Autodesk Inventor part; units mm, degrees
ref_plane "YZ Plane" through (0, 0, 0) normal (1, 0, 0) x (0, 1, 0)
ref_plane "XZ Plane" through (0, 0, 0) normal (0, 1, 0) x (-1, 0, 0)
ref_plane "XY Plane" through (0, 0, 0) normal (0, 0, 1) x (1, 0, 0)
sketch "Sketch1" plane through (0, 0, 0) normal (0, 0, 1) x (1, 0, 0)
  circle A0 centre (0, 0) radius 235
  circle A1 centre (0, 0) radius 275
  circle A2 centre (0, 0) radius 255 construction
  line L0 (0, 275) -> (0, 235) construction
  point P0 (0, 255)
  dimension "d9" = 510
  dimension "d10" = 40
extrude "Plate1" add sketch "Sketch1" along normal blind 3
sketch "Sketch2" plane through (0, 0, 3) normal (0, 0, 1) x (1, 0, 0)
  circle A0 centre (0, 0) radius 235 construction
  circle A1 centre (0, 0) radius 275 construction
  line L0 (0, 275) -> (0, 235) construction
  circle A2 centre (0, 255) radius 9
  dimension "d3" = 18
extrude "Extrusion1" cut sketch "Sketch2" against normal through all
pattern_circular "Circular Pattern1" count 16 over 360 about axis through (0, 0, 0) along (0, 0, 1) of "Extrusion1"
equation "\"d9\" = Шпил_пласт_диам_центров"
equation "\"d10\" = Шпил_пласт_ширина"
equation "\"d2\" = Thickness"
equation "\"BendRadius\" = Thickness"
equation "\"BendReliefWidth\" = Thickness"
equation "\"BendReliefDepth\" = 0.5 * Thickness"
equation "\"CornerReliefSize\" = 4 * Thickness"
equation "\"MinimumRemnant\" = 2 * Thickness"
equation "\"TransitionRadius\" = BendRadius"
equation "\"JacobiRadiusSize\" = BendRadius"
equation "\"GapSize\" = Thickness"
properties part number "ДМС 090 прокладка лицо"
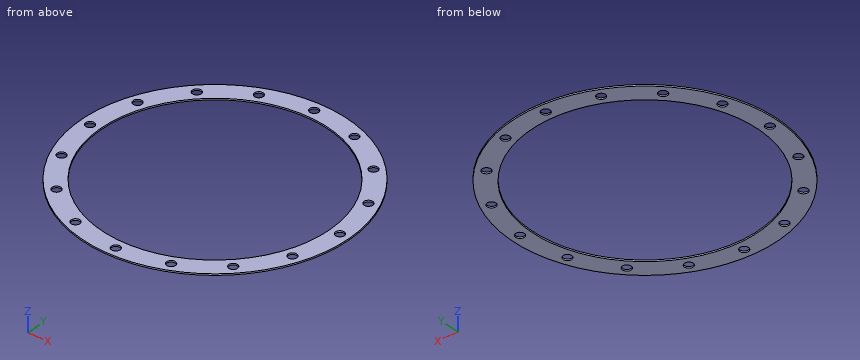
Part model, mm, in its own coordinate system. Round coordinates to 2 decimals unless told otherwise and drop trailing zeros. Order: outer loops, then holes, each group sorted by start corner. A loop starts at its lowest first (then second) coordinate and runs counter-clockwise, first axis right, second up. Notation, with made-up numbers: M 54.5,-18 L 90.5,-18 A26 cw 90.5,8 Z; hole C 62,13 d11. An arc over 180 degrees is marked long. Answer in a Markdown table with one row per item. Add a question column.
Q1. Pin check, flat tips, straight feed: pin 1 (20.5 mm diameter, centred on x = -255, y = 0, fed in from -Z); pin 2 (1 mm diameter, centred on x = -215.5, z = 2, fed in from +Y). Stop position of each tip, or through.
Q2. Wall check: L1, parallel to Y at x = 0, z = 2.25; L2, parallel to Y at x = 89.5, z = 2.7; L3, parallel to X at y = -243.5, z = 1.3. Give the ranges that are in metal, low to high. Write a range as from..to.
Q3. Cut at A-A on x = 0. Give the cut face in (y, z).
Q4. Cut at D-D on x = 255. Give the cut face in (y, z), and give its area (3 significant figures).
Q5. Cut at C-C on z = 1.35. Give the number of separate pieces and of enclosed holes in the cut face, and give its area (3 significant figures).
Q6. Cut at B-B on y = -43.5. Give the cut face in (x, z).
Established:
| question | item | result |
|---|---|---|
| 1 | pin 1 | stops at z = 0 |
| 1 | pin 2 | stops at y = 171.46 |
| 2 | L1 | y = -275..-264, -246..-235, 235..246, 264..275 |
| 2 | L2 | y = -260.03..-239.54, -231.63..-217.29, 217.29..231.63, 239.54..260.03 |
| 2 | L3 | x = -127.8..-101.88, -93.29..93.29, 101.88..127.8 |
| 3 | outline | M -275,0 L -264,0 L -264,3 L -275,3 Z; M -246,0 L -235,0 L -235,3 L -246,3 Z; M 235,0 L 246,0 L 246,3 L 235,3 Z; M 264,0 L 275,0 L 275,3 L 264,3 Z |
| 4 | outline | M -102.96,0 L -9,0 L -9,3 L -102.96,3 Z; M 9,0 L 102.96,0 L 102.96,3 L 9,3 Z |
| 4 | area | 564 mm2 |
| 5 | separate pieces | 1 |
| 5 | enclosed holes | 17 |
| 5 | area | 60,000 mm2 |
| 6 | outline | M -271.54,0 L -230.94,0 L -230.94,3 L -271.54,3 Z; M 230.94,0 L 271.54,0 L 271.54,3 L 230.94,3 Z |
